Verification items for the finished model (mm, model axes). Coordinates: 2 decimals unless noted, no trailing zeros. Order: outer loops, then holes, each group sorted by start corner. A loop starts at its lowest first (then second) coordinate and runs counter-clockwise, first axis right, second up. Notation, with made-up numbers: M 62,-22.75 L 101,-22.75 A13 ccw 101,-14.75 Z; hole C 84,14.5 d10. An arc over 180 degrees is marked long. Return JSON: item names as keys, results as strings. Group by question number.
Q1. Section check A-A, the plane x = -34. Enter the section's corners in (y, z).
Q2. Section check B-B, the plane y = -0.5. Enter the section's corners in (x, z).
Q3. Go/stop test with a flat-tipped pin: pin 1 Ø2 at (x, z) = (-39.5, 11.5) entering from -Y. Record where the tip stops, or that it passes through.
Q4. Thickness scan on probe 1 along X at (y, z) = (-0.3, 7); probe 2 along Z at (x, y) = (-40.5, -0.4); probe 3 along X at (y, z) = (-1.1, 0). Record the ranges inside material, lowest first.
Q5. Mould release check, pull along X, two halves, no side actions. Record for faces 1 (the face through (-47.622, -0.776, 4.186)), 2 (the face through (-32.76, -1, 11.87)), 3 (the face through (-17.43, -0.776, 4.186)): pulls with the +X half, pulls with the -X half, needs draft (parallel to the pull), parting line crosses it, or undercut.
from build123d import *

# Parameters (mm, degrees)
F0_W        = 44.4469191134
F0_H        = 30.4321236908
F1_DEPTH    = 2.032
F2_T1_DEPTH = 70.5752182711
F2_T3_DEPTH = 56.5604228486
F3_T1_DEPTH = 60.6284503053
F3_T3_DEPTH = 46.6136548828


# Not quite as in the source:
# - a fillet or chamfer that OpenCascade refuses, or shapes differently, is made with other operations: its cross-section is extruded or revolved along the edge and cut away or added
# - a feature of the source that left no trace in its solid (it failed there, or was rolled back) is left out


with BuildPart() as f1:
    # F0 (on Front) → F1 (new body)
    with BuildSketch(Plane.XZ):
        with Locations((-32.5259137899, 4.3256785721)):
            Rectangle(F0_W, F0_H)
    extrude(amount=F1_DEPTH)

    # F2: chamfer of 5.08 on 4 edges, made by hand

    # F2_s2 → F2_t1 (cut)
    with BuildSketch(Plane.YZ.offset(-67.8135229254)):
        Polygon((3.048, 19.5417404175), (-2.032, 14.4617404175), (-2.032, 19.5417404175), align=None)
        Polygon((3.048, -10.8903832734), (-2.032, -5.8103832734), (-2.032, -10.8903832734), align=None)
    extrude(amount=F2_T1_DEPTH, mode=Mode.SUBTRACT)

    # F2_s4 → F2_t3 (cut)
    with BuildSketch(Plane.XY.offset(-23.9545328522)):
        Polygon((-54.7493733466, 3.048), (-49.6693733466, -2.032), (-54.7493733466, -2.032), align=None)
        Polygon((-10.3024542332, 3.048), (-15.3824542332, -2.032), (-10.3024542332, -2.032), align=None)
    extrude(amount=F2_T3_DEPTH, mode=Mode.SUBTRACT)

    # F3: chamfer of 5.08 on 4 edges, made by hand

    # F3_s2 → F3_t1 (cut)
    with BuildSketch(Plane.YZ.offset(-62.8401389426)):
        Polygon((1.5601024484, -9.4024857218), (-2.032, -0.7303832734), (-2.032, -5.8103832734), align=None)
        Polygon((1.5601024484, 18.0538428659), (-2.032, 9.3817404175), (-2.032, 14.4617404175), align=None)
    extrude(amount=F3_T1_DEPTH, mode=Mode.SUBTRACT)

    # F3_s4 → F3_t3 (cut)
    with BuildSketch(Plane.XY.offset(-18.9811488694)):
        Polygon((-53.261475795, 1.5601024484), (-44.5893733466, -2.032), (-49.6693733466, -2.032), align=None)
        Polygon((-11.7903517848, 1.5601024484), (-20.4624542332, -2.032), (-15.3824542332, -2.032), align=None)
    extrude(amount=F3_T3_DEPTH, mode=Mode.SUBTRACT)


solid = f1.part
Numbers:
{
 "1": {"outline": "M -2.03,-0.73 L 0,-5.64 L 0,14.29 L -2.03,9.38 Z"},
 "2": {"outline": "M -48.29,-4.43 L -16.76,-4.43 L -16.76,13.08 L -48.29,13.08 Z"},
 "3": {"pin 1": "stops at y = -1.57"},
 "4": {"probe 1": "x = -48.77 to -16.28", "probe 2": "z = -4.67 to 13.32", "probe 3": "x = -46.84 to -18.21"},
 "5": {"face 1": "pulls with the -X half", "face 2": "needs draft", "face 3": "pulls with the +X half"}
}
